The listing builds one solid part. Answer for the finished solid, in the listing's coordinates (mm). Face numbers are marked on the shaded views. A direction names the side the tool comes from. Coordinates: 2 decimals unless noted, no trailing zeros. Write each loop counter-clockwise with the first axis right and the second up, starting at its lowest first coordinate (ties: lowest second). Pieces come first, ordered by that corner, then holes.
(1) The part is cut by section D-D on z = -1. Determine the outline of the cut face in (x, y), plus the area to 3 significant figures.
(2) For a pull along X with two mould halves and no side action, classify the marked faces 1, 2 and 3 as +X half, -X half, draft (parallel to the pull), parting line (faces both ways), or undercut.
(3) Given P1, Ø1, axis at y = 4.5, z = 0.5, coming from the +X side; P2, Ø1.1, axis at x = 1.5, y = 1.5, coming from the +Z side; P3, Ø2.5, axis at y = 1.5, z = -0.5, coming from the -X side, each flat-ended and moving along its own axis, determine where each tip first touches the part or whether it passes through.
(4) Straight lines are drawn through the part: line 1 (X direction, y = 4.65, z = 1); line 2 (Z direction, x = -0.75, y = 3.1); line 3 (Y direction, x = 4.25, z = 5.25). For each, find the intervals that lie inside material, in ascending order.
(5) The part is cut by section C-C on y = 1.5. Determine the outline of the cut face in (x, z).
(6) The part is cut by section A-A on y = 4.45. Determine the outline of the cut face in (x, z), plus the area to 3 significant figures.
(7) The part is cut by section B-B on x = 0.5. Determine the outline of the cut face in (y, z).
(8) Which of the six approach directions +Z, -Z, +X, -X, +Y, -Y give full straight-line access (tool end or side, diameter ignored) to the marked faces 4, 5, 6 and 7?
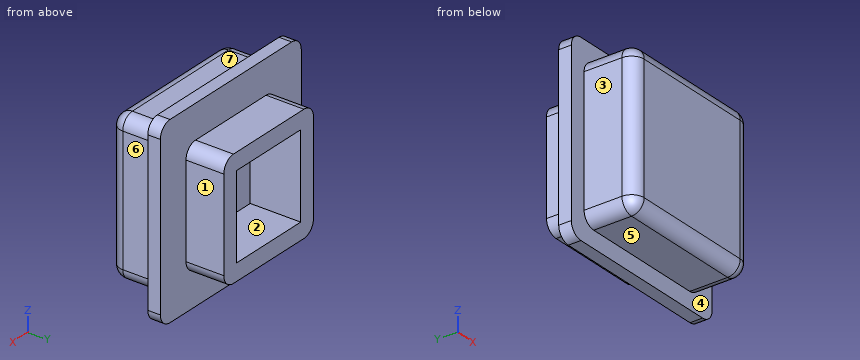
from build123d import *

# Parameters (mm, degrees)
SKETCH1_W           = 9
SKETCH1_H           = 9
BOSS_EXTRUDE1_DEPTH = 3
SKETCH2_W           = 11
SKETCH2_H           = 11
BOSS_EXTRUDE2_DEPTH = 0.75
SKETCH3_W           = 7
SKETCH3_H           = 7
SKETCH3_W_2         = 5
SKETCH3_H_2         = 5
BOSS_EXTRUDE3_DEPTH = 2.25
FILLET1_R           = 0.75
FILLET2_R           = 0.75
SKETCH4_W           = 5
SKETCH4_H           = 5
CUT_EXTRUDE1_DEPTH  = 0.75


with BuildPart() as part:
    # Sketch1 → Boss-Extrude1 (new body)
    with BuildSketch(Plane(origin=(0, 0, 0), x_dir=(1, 0, 0), z_dir=(0, 1, 0))):
        Rectangle(SKETCH1_W, SKETCH1_H)
    extrude(amount=BOSS_EXTRUDE1_DEPTH)

    # Sketch2 → Boss-Extrude2 (add)
    with BuildSketch(Plane(origin=(0, 3, 0), x_dir=(1, 0, 0), z_dir=(0, 1, 0))):
        Rectangle(SKETCH2_W, SKETCH2_H)
    extrude(amount=BOSS_EXTRUDE2_DEPTH)

    # Sketch3 → Boss-Extrude3 (add)
    with BuildSketch(Plane(origin=(0, 3.75, 0), x_dir=(1, 0, 0), z_dir=(0, 1, 0))):
        Rectangle(SKETCH3_W, SKETCH3_H)
        Rectangle(SKETCH3_W_2, SKETCH3_H_2, mode=Mode.SUBTRACT)
    extrude(amount=BOSS_EXTRUDE3_DEPTH)

    # Fillet1
    fillet1_edges = [part.edges().sort_by_distance(p)[0] for p in [
        (-5.5, 3.375, 5.5),
        (5.5, 3.375, 5.5),
        (5.5, 3.375, -5.5),
        (-5.5, 3.375, -5.5),
        (-3.5, 4.875, -3.5),
        (-3.5, 4.875, 3.5),
        (3.5, 4.875, 3.5),
        (3.5, 4.875, -3.5),
        (4.5, 1.5, 4.5),
        (-4.5, 1.5, 4.5),
        (-4.5, 1.5, -4.5),
        (4.5, 1.5, -4.5),
    ]]
    fillet(fillet1_edges, radius=FILLET1_R)

    # Fillet2
    fillet2_edges = [part.edges().sort_by_distance(p)[0] for p in [
        (0, 0, -4.5),
        (4.5, 0, 0),
        (0, 0, 4.5),
        (-4.5, 0, 0),
        (4.280330086, 0, 4.280330086),
        (-4.280330086, 0, 4.280330086),
        (-4.280330086, 0, -4.280330086),
        (4.280330086, 0, -4.280330086),
    ]]
    fillet(fillet2_edges, radius=FILLET2_R)

    # Sketch4 → Cut-Extrude1 (cut)
    with BuildSketch(Plane(origin=(0, 3.75, 0), x_dir=(1, 0, 0), z_dir=(0, 1, 0))):
        Rectangle(SKETCH4_W, SKETCH4_H)
    extrude(amount=-CUT_EXTRUDE1_DEPTH, mode=Mode.SUBTRACT)


solid = part.part
Model answer:
1. outline: (-5.5, 3) - (-4.5, 3) - (-4.5, 0.75) arc R0.75 ccw to (-3.75, 0) - (3.75, 0) arc R0.75 ccw to (4.5, 0.75) - (4.5, 3) - (5.5, 3) - (5.5, 3.75) - (3.5, 3.75) - (3.5, 6) - (2.5, 6) - (2.5, 3) - (-2.5, 3) - (-2.5, 6) - (-3.5, 6) - (-3.5, 3.75) - (-5.5, 3.75) - close
1. area: 35.8 mm2
2. face 1: +X half
2. face 2: undercut
2. face 3: -X half
3. P1: stops at x = 3.5
3. P2: stops at z = 4.5
3. P3: stops at x = -4.5
4. line 1: x = -3.5 to -2.5, 2.5 to 3.5
4. line 2: z = -5.5 to -2.5, 2.5 to 5.5
4. line 3: y = 3 to 3.75
5. outline: (-4.5, -3.75) arc R0.75 ccw to (-3.75, -4.5) - (3.75, -4.5) arc R0.75 ccw to (4.5, -3.75) - (4.5, 3.75) arc R0.75 ccw to (3.75, 4.5) - (-3.75, 4.5) arc R0.75 ccw to (-4.5, 3.75) - close
6. outline: (-3.5, -2.75) arc R0.75 ccw to (-2.75, -3.5) - (2.75, -3.5) arc R0.75 ccw to (3.5, -2.75) - (3.5, 2.75) arc R0.75 ccw to (2.75, 3.5) - (-2.75, 3.5) arc R0.75 ccw to (-3.5, 2.75) - close; hole (-2.5, -2.5) - (2.5, -2.5) - (2.5, 2.5) - (-2.5, 2.5) - close
6. area: 23.5 mm2
7. outline: (0, -3.75) arc R0.75 ccw to (0.75, -4.5) - (3, -4.5) - (3, -5.5) - (3.75, -5.5) - (3.75, -3.5) - (6, -3.5) - (6, -2.5) - (3, -2.5) - (3, 2.5) - (6, 2.5) - (6, 3.5) - (3.75, 3.5) - (3.75, 5.5) - (3, 5.5) - (3, 4.5) - (0.75, 4.5) arc R0.75 ccw to (0, 3.75) - close
8. face 4: -Y
8. face 5: -Z, +X, -X, -Y
8. face 6: +Z, -Z, +X, -Y
8. face 7: +Z, +X, -X, -Y
